from build123d import *

# Parameters (mm, degrees)
F0_W     = 9
F0_H     = 2.69917
F0_H_2   = 1.5
F1_DEPTH = 15
F2_R     = 1.55
F3_R     = 5
F4_SIZE  = 0.4


with BuildPart() as f1:
    # F0 (on Top) → F1 (new body)
    with BuildSketch(Plane.XY):
        Polygon((-9, -32), (-9, -29.30083), (-13.436408, -28.483649), (-13.917276, -31.094244), (-11.458638, -31.547122), align=None)
        with Locations((-4.5, -30.650415)):
            Rectangle(F0_W, F0_H)
        Polygon((-9, -33.5), (-9, -32), (-9.197668, -33.5), align=None)
        with Locations((-4.5, -32.75)):
            Rectangle(F0_W, F0_H_2)
        Polygon((-11.576222, -32.439408), (-11.458638, -31.547122), (-13.917276, -31.094244), align=None)
        with BuildLine():
            Line((0, -29.30083), (0, 29.30083))
            Line((0, 29.30083), (-9, 29.30083))
            ThreePointArc((-9, 29.30083), (-2.96804, 0), (-9, -29.30083))
            Line((-9, -29.30083), (0, -29.30083))
        make_face()
        with Locations((-4.5, 30.650415)):
            Rectangle(F0_W, F0_H)
        Polygon((0, 32), (0, 33.5), (-8.643575, 33.5), (-9, 32), align=None)
        Polygon((-9, 29.30083), (-9, 32), (-11.458638, 32.452878), (-13.917276, 32.905756), (-14.398145, 30.295161), align=None)
        Polygon((-13.917276, 32.905756), (-11.458638, 32.452878), (-11.250576, 33.328498), align=None)
    extrude(amount=F1_DEPTH)

    # F2
    f2_edges = [f1.edges().sort_by_distance(p)[0] for p in [
        (-14.398145, 30.295161, 7.5),
        (-9, 29.30083, 7.5),
        (-13.436408, -28.483649, 7.5),
        (-9, -29.30083, 7.5),
        (-13.917276, -31.094244, 7.5),
        (-13.917276, 32.905756, 7.5),
    ]]
    fillet(f2_edges, radius=F2_R)

    # F3
    f3_edges = [f1.edges().sort_by_distance(p)[0] for p in [
        (0, 33.5, 7.5),
        (0, -33.5, 7.5),
    ]]
    fillet(f3_edges, radius=F3_R)

    # F4
    f4_edges = [f1.edges().sort_by_distance(p)[0] for p in [
        (-7.098834, -33.5, 15),
        (-1.464466, -32.035534, 15),
        (-9.098834, -32.75, 15),
        (0, 0, 15),
        (-10.229319, -31.773561, 15),
        (-1.464466, 32.035534, 15),
        (-11.51743, -31.993265, 15),
        (-6.821787, 33.5, 15),
        (-12.271362, -32.039982, 15),
        (-8.821787, 32.75, 15),
        (-13.60087, -30.94777, 15),
        (-10.229319, 32.226439, 15),
        (-13.717913, -30.011919, 15),
        (-11.354607, 32.890688, 15),
        (-13.072174, -29.012362, 15),
        (-12.042412, 33.202971, 15),
        (-11.069446, -28.91964, 15),
        (-13.673826, 32.656158, 15),
        (-9.203231, -28.9109, 15),
        (-14.116639, 31.823431, 15),
        (-2.968333, 0.208446, 15),
        (-13.869431, 30.659395, 15),
        (-9.128357, 29.133809, 15),
        (-11.347475, 29.733232, 15),
        (-7.098834, -33.5, 0),
        (-1.464466, -32.035534, 0),
        (-9.098834, -32.75, 0),
        (0, 0, 0),
        (-10.229319, -31.773561, 0),
        (-1.464466, 32.035534, 0),
        (-11.51743, -31.993265, 0),
        (-6.821787, 33.5, 0),
        (-12.271362, -32.039982, 0),
        (-8.821787, 32.75, 0),
        (-13.60087, -30.94777, 0),
        (-10.229319, 32.226439, 0),
        (-13.717913, -30.011919, 0),
        (-11.354607, 32.890688, 0),
        (-13.072174, -29.012362, 0),
        (-12.042412, 33.202971, 0),
        (-11.069446, -28.91964, 0),
        (-13.673826, 32.656158, 0),
        (-9.203231, -28.9109, 0),
        (-14.116639, 31.823431, 0),
        (-2.968333, 0.208446, 0),
        (-13.869431, 30.659395, 0),
        (-9.128357, 29.133809, 0),
        (-11.347475, 29.733232, 0),
    ]]
    chamfer(f4_edges, length=F4_SIZE)


solid = f1.part
Source: CAD feature listing. Evaluate the final solid. Frame: model axes, mm. A direction names the side the tool comes from. Coordinates: 2 decimals unless noted, no trailing zeros.
Item 1: Set-up query: faces 4 (the face through (-8.82, 32.76, 7.4)), 5 (the face through (-13.66, 32.67, 7.6)), 6 (the face through (-9.137, 29.141, 7.599)). Return all of +Z, -Z, +X, -X, +Y, -Y with unobstructed straight access to the full face (end or side cutting, diameter ignored); none if empty.
Output values:
face 4: +Z, -Z, +Y
face 5: +Z, -Z, -X, +Y
face 6: +Z, -Z, -X
Item 2: Pull-direction query (X, two-part tool) for faces 1 (the face through (-12.335, -31.77, 14.803)), 2 (the face through (-9.097, -32.74, 7.401)), 3 (the face through (-7, -33.5, 7)); classes: pulls with the +X half, pulls with the -X half, needs draft (parallel to the pull), parting line crosses it, or undercut.
Output values:
face 1: pulls with the -X half
face 2: undercut
face 3: needs draft
Item 3: Material intervals for line 1 (Y direction, x = -11, z = 11.5); line 2 (X direction, y = -3.5, z = 5.5); line 3 (X direction, y = 27.5, z = 11.75), sorted ascending.
Output values:
line 1: y = -31.63 to -28.93, 29.67 to 32.37
line 2: x = -3.05 to 0
line 3: x = -8.25 to 0
Item 4: First-contact query: P1, Ø1, axis at y = 17, z = 6, coming from the -X side. Flat tip, straight axial feed; report the tip coordinate or a pass-through.
Output values:
P1: stops at x = -5.06
